Autodesk Inventor part; units mm, degrees
ref_plane "YZ Plane" through (0, 0, 0) normal (1, 0, 0) x (0, 1, 0)
ref_plane "XZ Plane" through (0, 0, 0) normal (0, 1, 0) x (-1, 0, 0)
ref_plane "XY Plane" through (0, 0, 0) normal (0, 0, 1) x (1, 0, 0)
sketch "Sketch1" plane through (0, 0, 0) normal (0, 1, 0) x (-1, 0, 0)
  line L0 (-1.35, 11.55) -> (-1.35, -11.55)
  line L1 (1.35, -11.55) -> (1.35, 11.55)
  arc A0 (1.35, 11.55) -> (-1.35, 11.55) centre (0, 11.55) ccw
  arc A1 (-1.35, -11.55) -> (1.35, -11.55) centre (0, -11.55) ccw
  line L2 (0, 12.9) -> (0, -12.9) construction
  point P0 (0, 0)
  point P1 (0, 0)
  dimension "d0" = 2.7
  dimension "d2" = 25.8
extrude "Extrusion1" add sketch "Sketch1" along normal blind 7
sketch "Sketch2" plane through (0, 7, 0) normal (0, 1, 0) x (1, 0, 0)
  line L0 (0.35, -11.55) -> (0.35, 11.55)
  line L1 (-0.35, 11.55) -> (-0.35, -11.55)
  arc A0 (-0.35, -11.55) -> (0.35, -11.55) centre (0, -11.55) ccw
  arc A1 (0.35, 11.55) -> (-0.35, 11.55) centre (0, 11.55) ccw
  line L2 (0, -11.9) -> (0, 11.9) construction
  point P0 (0, 0)
  point P1 (0, 0)
  dimension "d5" = 23.8
  dimension "d6" = 0.7
extrude "Extrusion2" cut sketch "Sketch2" against normal blind 6
chamfer "Chamfer1" distance 0.5 angle 45 4 edges at (1.35, 0, 0) (0, 0, -12.9) (-1.35, 0, 0) (0, 0, 12.9)
chamfer "Chamfer2" distance 0.5 angle 45 4 edges at (-0.35, 7, 0) (0, 7, -11.9) (0.35, 7, 0) (0, 7, 11.9)
equation "\"d5\" = pinlength"
equation "\"d6\" = pinwidth"
equation "\"d7\" = pinheight"
equation "\"pinwidth\" = 0.7"
equation "\"pinheight\" = 6"
equation "\"pinlength\" = 23.8"
properties part number "pin_header_protector"
Can you work these out from the model? Positions are in its coordinate system, mm. A direction names the side the tool comes from. Round coordinates to 2 decimals unless told otherwise and drop trailing zeros. Write each loop counter-clockwise with the first axis right and the second up, starting at its lowest first coordinate (ties: lowest second). Pieces come first, ordered by that corner, then holes. Notation, with made-up numbers: (-35.75, -10) -> (16.25, -10) arc R17 cw to (16.25, 1) -> close; hole circle Ø3 at (39.5, 13.5). An arc over 180 degrees is marked (long way). Use one line per item in the form item = value. Start each with the question number.
Q1. Imagine slicing it at C-C (z = -9.5). Please give me the cut outline in (x, y), then the cut area to 3 significant figures.
Q2. If I drill on probe 1 along X at (y, z) = (6.25, -6.75); probe 2 along Z at (x, y) = (0.05, 1.75); probe 3 along X at (y, z) = (6.75, -11.25), over which ranges is the centre line in solid material (lowest first)? Write a range as [from, to].
Q3. Which directions (+Z, -Z, +X, -X, +Y, -Y) give clear straight access to the entire face, cutting with the end or side of a thin tool? Please do faces 1 (the face through (0.01, 6.64, -12.04)), 2 (the face through (1.35, 4, 0)).
Q4. We'd pull the mould along Z, two halves only. Please class faces 3 (the face through (0, 0, 0)), 4 (the face through (0, 3.7, -12.9)), 5 (the face through (-0.35, 4, 0)): +Z half, -Z half, draft (parallel to the pull), parting line (faces both ways), or undercut.
Q5. Imagine slicing it at A-A (y = 4). Please give me the cut outline in (x, z), then the cut area to 3 significant figures.
Q6. Imagine slicing it at B-B (x = 0). Please give me the cut outline in (y, z), then the cut area to 3 significant figures.
Worked out:
q1.outline = (-1.35, 0.5) -> (-0.85, 0) -> (0.85, 0) -> (1.35, 0.5) -> (1.35, 7) -> (0.85, 7) -> (0.35, 6.5) -> (0.35, 1) -> (-0.35, 1) -> (-0.35, 6.5) -> (-0.85, 7) -> (-1.35, 7) -> close
q1.area = 14.2 mm^2
q2.probe_1 = [-1.35, -0.35], [0.35, 1.35]
q2.probe_2 = [-12.9, -11.9], [11.9, 12.9]
q2.probe_3 = [-1.35, -0.6], [0.6, 1.35]
q3.face_1 = +Y
q3.face_2 = +Z, -Z, +X, +Y, -Y
q4.face_3 = draft
q4.face_4 = -Z half
q4.face_5 = undercut
q5.outline = (-1.35, -11.55) arc R1.35 ccw to (1.35, -11.55) -> (1.35, 11.55) arc R1.35 ccw to (-1.35, 11.55) -> close; hole (-0.35, -11.55) arc R0.35 ccw to (0.35, -11.55) -> (0.35, 11.55) arc R0.35 ccw to (-0.35, 11.55) -> close
q5.area = 51.5 mm^2
q6.outline = (0, -12.4) -> (0.5, -12.9) -> (7, -12.9) -> (7, -12.4) -> (6.5, -11.9) -> (1, -11.9) -> (1, 11.9) -> (6.5, 11.9) -> (7, 12.4) -> (7, 12.9) -> (0.5, 12.9) -> (0, 12.4) -> close
q6.area = 37.3 mm^2
